Could you check a few things on this model? Use its own coordinates, in mm. A direction names the side the tool comes from. Give positions to 0.01 mm unless a question says otherwise; leave off trailing zeros. Write each loop counter-clockwise with the first axis right and the second up, starting at its lowest first coordinate (ties: lowest second). Pieces come first, ordered by that corner, then holes. Notation, with made-up numbers: (42, 24.25) - (63, 24.25) arc R13 cw to (63, 48.25) - close; hole circle Ø2 at (18.25, -30.5). An arc over 180 degrees is marked (long way). Use one line per item in the form item = value.
Autodesk Inventor part; units mm, degrees
ref_plane "Work Plane1" through (1.525, 0, 0) normal (0, 0, 1) x (1, 0, 0)
ref_plane "YZ Plane" through (0, 0, 0) normal (1, 0, 0) x (0, 1, 0)
ref_plane "XZ Plane" through (0, 0, 0) normal (0, 1, 0) x (-1, 0, 0)
sketch "Sketch1" plane through (0, 0, 0) normal (0, 0, 1) x (1, 0, 0)
  line L0 (0, 6.5) -> (0, 4)
  line L1 (3.7, 4) -> (25, 4)
  line L2 (25, 4) -> (25, 0)
  line L3 (25, 0) -> (-0.6001, 0)
  line L4 (-5.7201, 0) -> (30.12, 0)
  line L5 (-0.6001, 0) -> (-0.6001, 6.5)
  line L6 (-0.6001, 6.5) -> (0, 6.5)
  line L7 (3.7, 4) -> (2.9331, 4)
  line L8 (2.9331, 4) -> (0, 4)
  line L9 (0, -1.3) -> (0, 7.8)
  dimension "d0" = 25
  dimension "d1" = 21.3
  dimension "d2" = 8
  dimension "d9" = 0.6001
  dimension "d10" = 13
  dimension "d13" = 0.7669
  dimension "d14" = 8
revolve "Body" add sketch "Sketch1" angle 360 about axis through (25, 0, 0) along (-1, 0, 0)
sketch "Sketch2" plane through (-0.6001, 0, 0) normal (-1, 0, 0) x (0, 0, 1)
  line L0 (0, 7.5056) -> (6.5, 3.7528)
  line L1 (6.5, 3.7528) -> (6.5, -3.7528)
  line L2 (6.5, -3.7528) -> (0, -7.5056)
  line L3 (0, -7.5056) -> (-6.5, -3.7528)
  line L4 (-6.5, -3.7528) -> (-6.5, 3.7528)
  line L5 (-6.5, 3.7528) -> (0, 7.5056)
  point P0 (0, 0)
  point P1 (0, 0)
  dimension "d11" = 13
extrude "Head" add sketch "Sketch2" along normal blind 4.7
sketch "Sketch4" plane through (0, 0, 0) normal (0, 0, 1) x (1, 0, 0)
  line L0 (-5.3001, 6.5) -> (-5.3001, 7.5056)
  line L1 (-5.3001, 7.5056) -> (-4.7195, 7.5056)
  line L2 (-4.7195, 7.5056) -> (-5.3001, 6.5)
  line L3 (-6.2401, 0) -> (0.3399, 0)
  line L4 (-0.6001, 7.5056) -> (-5.3001, 7.5056)
  line L5 (-5.3001, 3.7528) -> (-5.3001, 7.5056)
  dimension "d5" = 30
  dimension "d19" = 13
revolve "Chamfer1" cut sketch "Sketch4" angle 360 about axis through (-10, 0, 0) along (1, 0, 0)
thread "Thread"
chamfer "Chamfer2" distance 0.7668 distance2 0.7669 1 edges at (25, -4, 0) measured on face at (25, 0.998, -0.8842)
ref_plane "Work Plane1" through (1.525, 0, 0) normal (0, 0, 1) x (1, 0, 0)
equation "\"d0\" = NLG"
equation "\"d1\" = GEL"
equation "\"d2\" = GD"
equation "\"d10\" = SD2"
equation "\"d14\" = BDM"
equation "\"d11\" = SW"
equation "\"d3\" = KOH - SD"
equation "\"d5\" = ANG1"
equation "\"d19\" = SW0"
equation "\"d15\" = GEL"
equation "\"d6\" = -0.5 * SPD + 0.5 * GD"
equation "\"NLG\" = 25"
equation "\"GD\" = NND"
equation "\"BDM\" = NND"
equation "\"KOH\" = 5.3"
equation "\"GEL\" = 21.3"
equation "\"SW\" = 13"
equation "\"SW0\" = SW"
equation "\"SPD\" = NND - 1.2269 * PTC"
equation "\"SD2\" = SW"
equation "\"SD\" = 0.6"
equation "\"ANG1\" = 30deg"
equation "\"GAL\" = 0.61345 * PTC"
equation "\"GUL\" = 0.61345 * PTC"
equation "\"RR\" = 0.4"
equation "\"WFT\" = SD"
equation "\"GD1\" = THREADDIA - 1.2269 * PTC"
equation "\"THREADDIA\" = 8"
equation "\"SDH\" = SW"
equation "\"TOA\" = 30deg"
equation "\"FAWI\" = 45deg"
equation "\"PTC\" = 1.25"
equation "\"NND\" = 8"
equation "\"E0\" = 1.155 * SW"
properties part number "AS 1110 - M8 x 25" material "Steel, Mild"
1. Imagine slicing it at A-A, the plane x = 5.5. List the corners of the cut face in (y, z) for me, and give its area (3 significant figures).
Response values:
outline = circle Ø8 at (0, 0)
area = 50.3 mm²
2. If I drill on line 1 (X direction, y = -3.75, z = -2.75); line 2 (Z direction, x = 10, y = 0); line 3 (Z direction, x = 9.5, y = 1.5), over which ranges is the centre line in solid material (lowest first)? Write a range as from..to.
Response values:
line_1 = -5.3..0
line_2 = -4..4
line_3 = -3.71..3.71
3. Which directions (+Z, -Z, +X, -X, +Y, -Y) give clear straight access to the entire face, cutting with the end or side of a thin tool? Please do faces 1 (the face through (-0.6, 7, 0)), 2 (the face through (-0.296, -5.158, -3.955)), 3 (the face through (-0.6, -7, 0)), 4 (the face through (-2.9, -5.6, 3.3)).
Response values:
face_1 = +X, +Y
face_2 = +X
face_3 = +X, -Y
face_4 = +Z, +X, -X, -Y
4. For pin 1 (2 mm diameter, centred on y = 3, z = -3.5, fed in from +X); pin 2 (2 mm diameter, centred on x = 7, z = 1.5, fed in from -Y); pin 3 (1 mm diameter, centred on x = 0, y = -2, fed in from -Z), each with a flat end and sliding along its axis, tell me the tip position at first contact or that it passes through.
Response values:
pin_1 = 24.62
pin_2 = -3.97
pin_3 = -6.32
